from build123d import *

# Parameters (mm, degrees)
SKETCH1_W           = 215
SKETCH1_H           = 145
BOSS_EXTRUDE1_DEPTH = 130
SKETCH3_W           = 30
SKETCH3_H           = 30
CUT_EXTRUDE1_DEPTH  = 262.498087947
SKETCH4_W           = 198
SKETCH4_H           = 125
CUT_EXTRUDE2_DEPTH  = 115
SKETCH5_W           = 34.065007978
SKETCH5_H           = 64.63018637
CUT_EXTRUDE3_DEPTH  = 115
SKETCH6_W           = 35
SKETCH6_H           = 80
CUT_EXTRUDE4_DEPTH  = 115
SKETCH7_W           = 60
SKETCH7_H           = 35
CUT_EXTRUDE5_DEPTH  = 115


with BuildPart() as part:
    # Sketch1 → Boss-Extrude1 (new body)
    with BuildSketch(Plane.XY):
        Rectangle(SKETCH1_W, SKETCH1_H)
    extrude(amount=BOSS_EXTRUDE1_DEPTH)

    # Sketch3 → Cut-Extrude1 (cut, through all)
    with BuildSketch(Plane.ZY.offset(107.5)):
        with Locations((15, -17.5)):
            Rectangle(SKETCH3_W, SKETCH3_H)
    extrude(amount=-CUT_EXTRUDE1_DEPTH, mode=Mode.SUBTRACT)

    # Sketch4 → Cut-Extrude2 (cut)
    with BuildSketch(Plane(origin=(0, 0, 0), x_dir=(-1, 0, 0), z_dir=(0, 0, -1))):
        Rectangle(SKETCH4_W, SKETCH4_H)
    extrude(amount=-CUT_EXTRUDE2_DEPTH, mode=Mode.SUBTRACT)

    # Sketch5 → Cut-Extrude3 (cut)
    with BuildSketch(Plane.XY.offset(130)):
        with Locations((-74.429709212, 4.666439449)):
            Rectangle(SKETCH5_W, SKETCH5_H)
    extrude(amount=-CUT_EXTRUDE3_DEPTH, mode=Mode.SUBTRACT)

    # Sketch6 → Cut-Extrude4 (cut)
    with BuildSketch(Plane.XY.offset(130)):
        with Locations((52.031651923, 6.984940898)):
            Rectangle(SKETCH6_W, SKETCH6_H)
    extrude(amount=-CUT_EXTRUDE4_DEPTH, mode=Mode.SUBTRACT)

    # Sketch7 → Cut-Extrude5 (cut)
    with BuildSketch(Plane.XZ.offset(72.5)):
        with Locations((2.5, 17.5)):
            Rectangle(SKETCH7_W, SKETCH7_H)
    extrude(amount=-CUT_EXTRUDE5_DEPTH, mode=Mode.SUBTRACT)


solid = part.part
Work out the finished part from the listing and answer in its coordinate system (mm). A direction names the side the tool comes from. Give positions to 0.01 mm unless a question says otherwise; leave off trailing zeros. Loops run counter-clockwise (first coordinate to the right, second up) from the corner with the lowest first, then second, coordinate; pieces in that order, holes last. Notation, with made-up numbers: (57.25, 6) -> (116.25, 6) arc R21 ccw to (116.25, 19) -> close; hole circle Ø8 at (-8, 64.5). An arc over 180 degrees is marked (long way). Use a Markdown table: item, result. Add a question column.
1. Find the intervals of material crossed by probe 1 along X at (y, z) = (-16, 121.5); probe 2 along Y at (x, z) = (87, 20.5); probe 3 along X at (y, z) = (-4, 47), in increasing order.
2. Determine the mould class of faces 4 (the flat face through (107.5, -1, 64)), 5 (the flat face through (-2, 72.5, 64)), 6 (the flat face through (2, -68, 35)) for opening direction X: released by +X, released by -X, zero draft, split by the parting line, or undercut.
3. Section C-C on y = -49 is taken. Determine the outline of the cut face in (x, z).
4. Flat-ended cylindrical pins translate along their axes: pin 1 Ø4 at (x, y) = (-101, -16.5) entering from -Z; pin 2 Ø4 at (x, y) = (42.5, 50.5) entering from -Z. Find the tip coordinate at first contact, or state that the pin passes through.
5. Section A-A on z = 62.5 is taken. Determine the outline of the cut face in (x, y), and give its area (4 significant figures).
6. Section B-B on x = -80 is taken. Determine the outline of the cut face in (y, z).
7. Section D-D on y = -6 is taken. Determine the outline of the cut face in (x, z).
8. For faces 1 (the flat face through (69.532, 6, 123)), 2 (the flat face through (-99, -1, 57)), 3 (the flat face through (103, -32.5, 15)), determine the directions among +Z, -Z, +X, -X, +Y, -Y from which every point of the face is accessible in a straight line to the end or side of a thin tool.
Results below:
| question | item | result |
|---|---|---|
| 1 | probe 1 | x = -107.5 to -91.46, -57.4 to 34.53, 69.53 to 107.5 |
| 1 | probe 2 | y = -72.5 to -62.5, 62.5 to 72.5 |
| 1 | probe 3 | x = -107.5 to -99, 99 to 107.5 |
| 2 | face 4 | released by +X |
| 2 | face 5 | zero draft |
| 2 | face 6 | undercut |
| 3 | outline | (-107.5, 0) -> (-99, 0) -> (-99, 115) -> (99, 115) -> (99, 0) -> (107.5, 0) -> (107.5, 130) -> (-107.5, 130) -> close |
| 4 | pin 1 | stops at z = 30 |
| 4 | pin 2 | stops at z = 115 |
| 5 | outline | (-107.5, -72.5) -> (107.5, -72.5) -> (107.5, 72.5) -> (-107.5, 72.5) -> close; hole (-99, -62.5) -> (99, -62.5) -> (99, 62.5) -> (-99, 62.5) -> close |
| 5 | area | 6,425 mm^2 |
| 6 | outline | (-72.5, 0) -> (-62.5, 0) -> (-62.5, 115) -> (-27.65, 115) -> (-27.65, 130) -> (-72.5, 130) -> close; (36.98, 115) -> (62.5, 115) -> (62.5, 0) -> (72.5, 0) -> (72.5, 130) -> (36.98, 130) -> close |
| 7 | outline | (-107.5, 30) -> (-99, 30) -> (-99, 115) -> (-91.46, 115) -> (-91.46, 130) -> (-107.5, 130) -> close; (-57.4, 115) -> (34.53, 115) -> (34.53, 130) -> (-57.4, 130) -> close; (69.53, 115) -> (99, 115) -> (99, 30) -> (107.5, 30) -> (107.5, 130) -> (69.53, 130) -> close |
| 8 | face 1 | +Z, -Z |
| 8 | face 2 | -Z |
| 8 | face 3 | -Z, +X, -X |
